```python
from build123d import *

# Parameters (mm, degrees)
SKETCH1_R           = 2.5
BOSS_EXTRUDE1_DEPTH = 20


with BuildPart() as part:
    # Sketch1 → Boss-Extrude1 (new body)
    with BuildSketch(Plane(origin=(0, 0, 0), x_dir=(1, 0, 0), z_dir=(0, 1, 0))):
        with BuildLine():
            Line((-16.572928834, 3.745367509), (-16.572928834, -16.254632491))
            Line((-16.572928834, -16.254632491), (18.427071166, -16.254632491))
            Line((18.427071166, -16.254632491), (18.427071166, 3.745367509))
            Line((18.427071166, 3.745367509), (6.415332466, 3.745367509))
            add(Edge.make_bspline(
                [(-3.819533202, 3.745367509), (1.198635577, 7.766174081), (6.415332466, 3.745367509)],
                knots=[0, 0, 0, 1, 1, 1], degree=2))
            Line((-3.819533202, 3.745367509), (-16.572928834, 3.745367509))
        make_face()
        with Locations((0.927071166, 0)):
            Circle(SKETCH1_R, mode=Mode.SUBTRACT)
    extrude(amount=BOSS_EXTRUDE1_DEPTH)


solid = part.part
```
Source: CAD feature listing. Evaluate the final solid. Frame: model axes, mm. A direction names the side the tool comes from. Give positions to 0.01 mm unless a question says otherwise; leave off trailing zeros. Loops run counter-clockwise (first coordinate to the right, second up) from the corner with the lowest first, then second, coordinate; pieces in that order, holes last. Notation, with made-up numbers: (60, -17) -> (113, -17) arc R27 cw to (113, 11) -> close; hole circle Ø1 at (24, -30). An arc over 180 degrees is marked (long way). Put each result on its own line as item: value. Start each with the question number.
1) Material intervals for probe 1 along X at (y, z) = (14.5, 0); probe 2 along Z at (x, y) = (1, 2); probe 3 along Z at (x, y) = (8, 17.25), sorted ascending.
2) Draft query along X for faces 4 (the face through (18.427, 10, 6)), 5 (the face through (1, 0, 7)), 6 (the face through (0.39, 9.86, 2.44)). Return one class per face: released by +X, released by -X, zero draft, split by the parting line, or undercut.
3) Contact query for a flat-ended pin moving along its axis: P1, Ø5, axis at x = -9, y = 6, coming from the -Z side. Output: stop coordinate, or through.
4) Cut plane A-A (z = 0). Return loops of the section in (x, y).
5) Cut plane B-B (x = -12). Return loops of the section in (y, z).
6) Reachability of faces 1 (the face through (-10, 10, -3.745)), 2 (the face through (1, 10, 16.255)), 3 (the face through (13, 10, -3.745)) from +Z, -Z, +X, -X, +Y, -Y: full face, straight path, thin tool, end or side. Return the list, or none.
Results are:
1. probe 1: x = -16.57 to -1.57, 3.43 to 18.43
1. probe 2: z = -5.75 to -2.5, 2.5 to 16.25
1. probe 3: z = -3.75 to 16.25
2. face 4: released by +X
2. face 5: zero draft
2. face 6: undercut
3. P1: stops at z = -3.75
4. outline: (-16.57, 0) -> (-1.57, 0) -> (-1.57, 20) -> (-16.57, 20) -> close; (3.43, 0) -> (18.43, 0) -> (18.43, 20) -> (3.43, 20) -> close
5. outline: (0, -3.75) -> (20, -3.75) -> (20, 16.25) -> (0, 16.25) -> close
6. face 1: -Z, -X, +Y, -Y
6. face 2: +Z, +X, -X, +Y, -Y
6. face 3: -Z, +X, +Y, -Y
